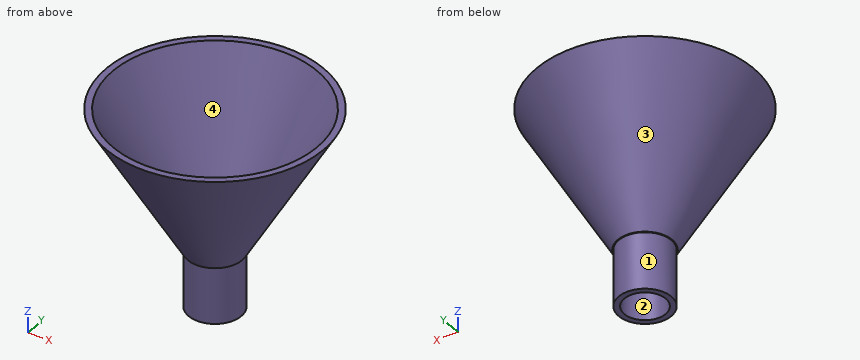
```python
from build123d import *

# Parameters (mm, degrees)
F0_R     = 2.8
F0_R_2   = 2.2
F1_DEPTH = 6


with BuildPart() as f1:
    # F0 (on Top) → F1 (new body)
    with BuildSketch(Plane.XY):
        Circle(F0_R)
        Circle(F0_R_2, mode=Mode.SUBTRACT)
    extrude(amount=F1_DEPTH)

    # F2 (on Front) → F3 (revolve)
    with BuildSketch(Plane.XZ):
        Polygon((10.860254, 21), (2.2, 6), (2.9, 6), (11.560254, 21), align=None)
    revolve(axis=Axis((0, 0, 15.443827), (0, 0, 1)))


solid = f1.part
```
Geometry check sheet. Reference: the model listing, model coordinates, mm. Face numbers are marked on the shaded views. A direction names the side the tool comes from. Round coordinates to 2 decimals unless told otherwise and drop trailing zeros. Order: outer loops, then holes, each group sorted by start corner. A loop starts at its lowest first (then second) coordinate and runs counter-clockwise, first axis right, second up. Notation, with made-up numbers: (75.5, -35.5) - (121.5, -35.5) arc R17 ccw to (121.5, -13.5) - close; hole circle Ø6 at (31.5, 52). An arc over 180 degrees is marked (long way). Use a Markdown table: item, result. Add a question column.
(1) Depth check by flat-ended pin: pin 1 (4.5 mm diameter, centred on x = 0.5, y = -1, fed in from -Z); pin 2 (8 mm diameter, centred on x = -4.5, y = 8.5, fed in from -Z); pin 3 (1 mm diameter, centred on x = 7, y = -1, fed in from +Z); pin 4 (10 mm diameter, centred on x = -2.5, z = 9, fed in from +Y). Enter the tip coordinate at first touch or a pass-through.
(2) Tool access check on the marked faces 1 and 2. Record the directions out of +Z, -Z, +X, -X, +Y, -Y that give a thin tool (end or side, any length) a straight path to the whole face; none if there is none.
(3) Release check for a two-part mould opening along X. For the marked faces 3 and 4 record: pulls with the +X half, pulls with the -X half, needs draft (parallel to the pull), parting line crosses it, or undercut.
(4) Sectioned sample at D-D, the plane z = 18.5. Enter the section's corners in (x, y), and give its area (3 significant figures).
(5) Sectioned sample at C-C, the plane z = 1.5. Enter the section's corners in (x, y), and give its area (3 significant figures).
(6) Material ranges on line 1 along Y through (x, z) = (0, 2.8); line 2 along Y through (x, z) = (6.25, 19.25); line 3 along X through (y, z) = (4, 15.75), recorded low to high. Write a range as [from, to].
(7) Sectioned sample at A-A, the plane x = 0. Enter the section's corners in (y, z), and give its area (3 significant figures).
Answers below:
| question | item | result |
|---|---|---|
| 1 | pin 1 | z = 0 |
| 1 | pin 2 | z = 10.71 |
| 1 | pin 3 | z = 15.3 |
| 1 | pin 4 | y = 7.32 |
| 2 | face 1 | -Z |
| 2 | face 2 | +Z, -Z |
| 3 | face 3 | parting line crosses it |
| 3 | face 4 | undercut |
| 4 | outline | circle Ø20.23 at (0, 0); hole circle Ø18.83 at (0, 0) |
| 4 | area | 43.0 mm² |
| 5 | outline | circle Ø5.6 at (0, 0); hole circle Ø4.4 at (0, 0) |
| 5 | area | 9.42 mm² |
| 6 | line 1 | [-2.8, -2.2], [2.2, 2.8] |
| 6 | line 2 | [-8.5, -7.61], [7.61, 8.5] |
| 6 | line 3 | [-7.53, -6.73], [6.73, 7.53] |
| 7 | outline | (-11.56, 21) - (-2.9, 6) - (-2.8, 6) - (-2.8, 0) - (-2.2, 0) - (-2.2, 6) - (-10.86, 21) - close; (2.2, 0) - (2.8, 0) - (2.8, 6) - (2.9, 6) - (11.56, 21) - (10.86, 21) - (2.2, 6) - close |
| 7 | area | 28.2 mm² |
